Geometry check sheet. Reference: the model listing, model coordinates, mm. Face numbers are marked on the shaded views. A direction names the side the tool comes from. Coordinates: 2 decimals unless noted, no trailing zeros. Order: outer loops, then holes, each group sorted by start corner. A loop starts at its lowest first (then second) coordinate and runs counter-clockwise, first axis right, second up.
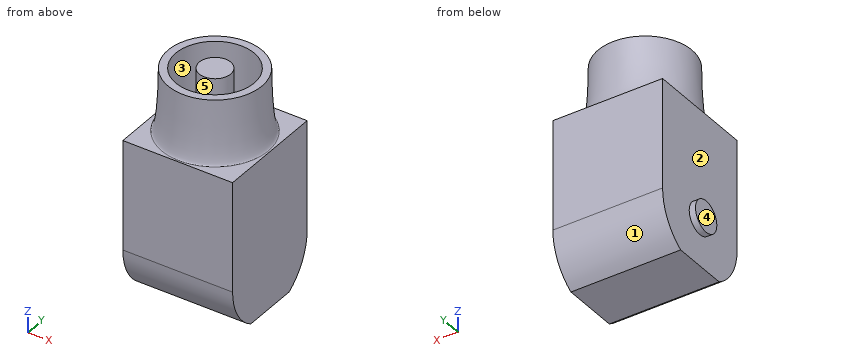
```python
from build123d import *

# Parameters (mm, degrees)
AUFSATZ_LINEAR_AUSTRAGEN1_DEPTH = 35
SKIZZE3_R                       = 14.969948268
SKIZZE3_R_2                     = 12.5
SKIZZE3_R_3                     = 5
AUFSATZ_LINEAR_AUSTRAGEN2_DEPTH = 20
VERRUNDUNG1_SIZE                = 2
VERRUNDUNG1_SIZE_2              = 20
SKIZZE4_R                       = 5
AUFSATZ_LINEAR_AUSTRAGEN3_DEPTH = 2


with BuildPart() as part:
    # Skizze2 → Aufsatz-Linear austragen1 (new body)
    with BuildSketch(Plane(origin=(0, 0, 0), x_dir=(0, 0, -1), z_dir=(1, 0, 0))):
        with BuildLine():
            Line((-35, -17.5), (3.5e-08, -17.5))
            ThreePointArc((3.5e-08, -17.5), (8.617050894, -15.231429148), (15, -9.013878189))
            Line((15, -9.013878189), (15, 9.013878189))
            ThreePointArc((15, 9.013878189), (8.61705092, 15.231429133), (9.5e-08, 17.5))
            Line((9.5e-08, 17.5), (-35, 17.5))
            Line((-35, 17.5), (-35, -17.5))
        make_face()
    extrude(amount=AUFSATZ_LINEAR_AUSTRAGEN1_DEPTH)

    # Skizze3 → Aufsatz-Linear austragen2 (add)
    # profile 1 of 2: a face of its own
    with BuildSketch(Plane.XY.offset(35)):
        with Locations(Location((17.5, 0, 0), (0, 0, 90))):
            Circle(SKIZZE3_R)
        with Locations((17.5, 0)):
            Circle(SKIZZE3_R_2, mode=Mode.SUBTRACT)
    # profile 2 of 2: a face of its own
    with BuildSketch(Plane.XY.offset(35)):
        with Locations(Location((17.5, 0, 0), (0, 0, 90))):
            Circle(SKIZZE3_R_3)
    extrude(amount=AUFSATZ_LINEAR_AUSTRAGEN2_DEPTH)

    # Verrundung1
    # an asymmetric fillet: 20, 2 mm, written as the material it adds along each edge
    with BuildSketch(Plane(origin=(17.5, 0, 35), x_dir=(0, 1, 0), z_dir=(1, 0, 0))) as verrundung1_piece_1:
        with BuildLine():
            Bezier((14.969948268 + VERRUNDUNG1_SIZE, 0), (14.969948268, 0), (14.969948268, VERRUNDUNG1_SIZE_2), weights=[1, 0.707106781, 1])
            Line((14.969948268, VERRUNDUNG1_SIZE_2), (14.969948268, 0))
            Line((14.969948268, 0), (14.969948268 + VERRUNDUNG1_SIZE, 0))
        make_face()
    revolve(axis=Axis((17.5, 0, 35), (0, 0, 1)))

    # Skizze4 → Aufsatz-Linear austragen3 (add)
    with BuildSketch(Plane.ZY):
        with Locations(Location((0, 0, 0), (0, 0, 180))):
            Circle(SKIZZE4_R)
    extrude(amount=AUFSATZ_LINEAR_AUSTRAGEN3_DEPTH)


solid = part.part
```
Item 1: Release check for a two-part mould opening along Y. For the marked faces 1, 2 and 3 record: pulls with the +Y half, pulls with the -Y half, needs draft (parallel to the pull), parting line crosses it, or undercut.
Item 2: Thickness scan on line 1 along Y through (x, z) = (13.5, 40.5); line 2 along Y through (x, z) = (17, 42); line 3 along Z through (x, y) = (17.5, -8). Record the ranges inside material, lowest first.
Item 3: Depth check by flat-ended pin: P1, Ø2, axis at y = -4, z = 7.5, coming from the -X side; P2, Ø6, axis at x = 5, z = 48, coming from the +Y side. Enter the tip coordinate at first touch or a pass-through.
Item 4: Sectioned sample at A-A (z = 10). Record the cut outline in (x, y).
Item 5: Tool access check on the marked faces 4 and 5. Record the directions out of +Z, -Z, +X, -X, +Y, -Y that give a thin tool (end or side, any length) a straight path to the whole face; none if there is none.
Geometry check:
1. face 1: pulls with the +Y half
1. face 2: needs draft
1. face 3: undercut
2. line 1: y = -15.07 to -11.84, -3 to 3, 11.84 to 15.07
2. line 2: y = -15.44 to -12.49, -4.97 to 4.97, 12.49 to 15.44
2. line 3: z = -15 to 35
3. P1: stops at x = 0
3. P2: stops at y = 11.74
4. outline: (0, -17.5) - (35, -17.5) - (35, 17.5) - (0, 17.5) - close
5. face 4: +Z, -Z, -X, +Y, -Y
5. face 5: +Z
